Autodesk Inventor part; units mm, degrees
ref_plane "YZ Plane" through (0, 0, 0) normal (1, 0, 0) x (0, 1, 0)
ref_plane "XZ Plane" through (0, 0, 0) normal (0, 1, 0) x (-1, 0, 0)
ref_plane "XY Plane" through (0, 0, 0) normal (0, 0, 1) x (1, 0, 0)
ref_plane "작업 평면1" through (44.8, 0, -17) normal (-1, 0, 0) x (0, 0, 1)
sketch "스케치2" plane through (44.8, 0, -17) normal (-1, 0, 0) x (0, 0, 1)
  arc A0 (-19.5808, 6.2636) -> (-20.1, 4.5766) centre (-17.1, 4.5766) ccw
  line L0 (-20.1, -39.6766) -> (-20.1, 4.5766)
  arc A1 (-20.1, -39.6766) -> (-19.5808, -41.3636) centre (-17.1, -39.6766) ccw
  line L1 (-15.8929, -46.7869) -> (-19.5808, -41.3636)
  arc A2 (-15.8929, -46.7869) -> (-13.4121, -48.1) centre (-13.4121, -45.1) ccw
  line L2 (13.4121, -48.1) -> (-13.4121, -48.1)
  arc A3 (13.4121, -48.1) -> (15.8929, -46.7869) centre (13.4121, -45.1) ccw
  line L3 (19.5808, -41.3636) -> (15.8929, -46.7869)
  arc A4 (19.5808, -41.3636) -> (20.1, -39.6766) centre (17.1, -39.6766) ccw
  line L4 (20.1, 4.5766) -> (20.1, -39.6766)
  arc A5 (20.1, 4.5766) -> (19.5808, 6.2636) centre (17.1, 4.5766) ccw
  line L5 (15.5953, 12.1246) -> (19.5808, 6.2636)
  arc A6 (15.5953, 12.1246) -> (13.9414, 13) centre (13.9414, 11) ccw
  line L6 (7.65, 13) -> (13.9414, 13)
  arc A7 (9.15, 11.5) -> (7.65, 13) centre (7.65, 11.5) ccw
  line L7 (9.15, 11.5) -> (9.15, 10)
  arc A8 (9.15, 10) -> (11.5, 7.65) centre (11.5, 10) ccw
  line L8 (11.5, 7.65) -> (13.5, 7.65)
  arc A9 (14.5, 6.65) -> (13.5, 7.65) centre (13.5, 6.65) ccw
  line L9 (14.5, 6.65) -> (14.5, -36.15)
  arc A10 (13.5, -37.15) -> (14.5, -36.15) centre (13.5, -36.15) ccw
  line L10 (13.5, -37.15) -> (11.5, -37.15)
  arc A11 (11.5, -37.15) -> (9.15, -39.5) centre (11.5, -39.5) ccw
  line L11 (9.15, -39.5) -> (9.15, -41.5)
  arc A12 (8.15, -42.5) -> (9.15, -41.5) centre (8.15, -41.5) ccw
  line L12 (8.15, -42.5) -> (-8.15, -42.5)
  arc A13 (-9.15, -41.5) -> (-8.15, -42.5) centre (-8.15, -41.5) ccw
  line L13 (-9.15, -41.5) -> (-9.15, -39.5)
  arc A14 (-9.15, -39.5) -> (-11.5, -37.15) centre (-11.5, -39.5) ccw
  line L14 (-11.5, -37.15) -> (-13.5, -37.15)
  arc A15 (-14.5, -36.15) -> (-13.5, -37.15) centre (-13.5, -36.15) ccw
  line L15 (-14.5, -36.15) -> (-14.5, 6.65)
  arc A16 (-13.5, 7.65) -> (-14.5, 6.65) centre (-13.5, 6.65) ccw
  line L16 (-13.5, 7.65) -> (-11.5, 7.65)
  arc A17 (-11.5, 7.65) -> (-9.15, 10) centre (-11.5, 10) ccw
  line L17 (-9.15, 10) -> (-9.15, 11.5)
  arc A18 (-7.65, 13) -> (-9.15, 11.5) centre (-7.65, 11.5) ccw
  line L18 (-13.9414, 13) -> (-7.65, 13)
  arc A19 (-13.9414, 13) -> (-15.5953, 12.1246) centre (-13.9414, 11) ccw
  line L19 (-19.5808, 6.2636) -> (-15.5953, 12.1246)
  circle A20 centre (17.3, 4) radius 1.35
  circle A21 centre (17.3, -18) radius 1.35
  circle A22 centre (11, -45.3) radius 1.35
  circle A23 centre (-17.3, 4) radius 1.35
  circle A24 centre (-17.3, -18) radius 1.35
  circle A25 centre (-11, -45.3) radius 1.35
  circle A26 centre (17.3, -40) radius 1.35
  circle A27 centre (-17.3, -40) radius 1.35
  line L20 (17.3, -19.35) -> (17.3, 5.35)
  line L21 (20.1, 4.5766) -> (20.1, 6.65)
  line L22 (20.1, 6.65) -> (14.5, 6.65)
  line L23 (17.3, -7) -> (20.1, -7)
  arc A28 (19.5808, -20.2636) -> (20.1, -18.5766) centre (17.1, -18.5766) ccw
  line L24 (20.1, -18.5766) -> (20.1, -20.65)
  line L25 (20.1, -20.65) -> (14.5, -20.65)
  line L26 (20.1, -20.65) -> (14.5, -20.65)
  line L27 (14.5, -20.65) -> (14.5, 6.65)
  line L28 (14.5, 6.65) -> (20.1, 6.65)
  line L29 (20.1, 6.65) -> (20.1, -20.65)
  line L30 (14.6, -36.15) -> (14.6, 6.65)
  arc A29 (14.6, 6.65) -> (13.5, 7.75) centre (13.5, 6.65) ccw
  line L31 (13.5, 7.75) -> (11.5, 7.75)
  arc A30 (9.25, 10) -> (11.5, 7.75) centre (11.5, 10) ccw
  line L32 (9.25, 10) -> (9.25, 11.5)
  arc A31 (9.25, 11.5) -> (8.4246, 12.9) centre (7.65, 11.5) ccw
  line L33 (8.4246, 12.9) -> (13.9414, 12.9)
  arc A32 (15.5126, 12.0684) -> (13.9414, 12.9) centre (13.9414, 11) ccw
  line L34 (15.5126, 12.0684) -> (19.4981, 6.2073)
  arc A33 (20, 4.5766) -> (19.4981, 6.2073) centre (17.1, 4.5766) ccw
  line L35 (20, 4.5766) -> (20, -39.6766)
  arc A34 (19.4981, -41.3073) -> (20, -39.6766) centre (17.1, -39.6766) ccw
  line L36 (19.4981, -41.3073) -> (15.8102, -46.7307)
  arc A35 (13.4121, -48) -> (15.8102, -46.7307) centre (13.4121, -45.1) ccw
  line L37 (13.4121, -48) -> (-13.4121, -48)
  arc A36 (-15.8102, -46.7307) -> (-13.4121, -48) centre (-13.4121, -45.1) ccw
  line L38 (-15.8102, -46.7307) -> (-19.4981, -41.3073)
  arc A37 (-20, -39.6766) -> (-19.4981, -41.3073) centre (-17.1, -39.6766) ccw
  line L39 (-20, -39.6766) -> (-20, 4.5766)
  arc A38 (-19.4981, 6.2073) -> (-20, 4.5766) centre (-17.1, 4.5766) ccw
  line L40 (-19.4981, 6.2073) -> (-15.5126, 12.0684)
  arc A39 (-13.9414, 12.9) -> (-15.5126, 12.0684) centre (-13.9414, 11) ccw
  line L41 (-13.9414, 12.9) -> (-8.4246, 12.9)
  arc A40 (-8.4246, 12.9) -> (-9.25, 11.5) centre (-7.65, 11.5) ccw
  line L42 (-9.25, 11.5) -> (-9.25, 10)
  arc A41 (-11.5, 7.75) -> (-9.25, 10) centre (-11.5, 10) ccw
  line L43 (-11.5, 7.75) -> (-13.5, 7.75)
  arc A42 (-13.5, 7.75) -> (-14.6, 6.65) centre (-13.5, 6.65) ccw
  line L44 (-14.6, 6.65) -> (-14.6, -36.15)
  arc A43 (-14.6, -36.15) -> (-13.5, -37.25) centre (-13.5, -36.15) ccw
  line L45 (-13.5, -37.25) -> (-11.5, -37.25)
  arc A44 (-9.25, -39.5) -> (-11.5, -37.25) centre (-11.5, -39.5) ccw
  line L46 (-9.25, -39.5) -> (-9.25, -41.5)
  arc A45 (-9.25, -41.5) -> (-8.15, -42.6) centre (-8.15, -41.5) ccw
  line L47 (-8.15, -42.6) -> (8.15, -42.6)
  arc A46 (8.15, -42.6) -> (9.25, -41.5) centre (8.15, -41.5) ccw
  line L48 (9.25, -41.5) -> (9.25, -39.5)
  arc A47 (11.5, -37.25) -> (9.25, -39.5) centre (11.5, -39.5) ccw
  line L49 (11.5, -37.25) -> (13.5, -37.25)
  arc A48 (13.5, -37.25) -> (14.6, -36.15) centre (13.5, -36.15) ccw
  line L50 (20, 4.5766) -> (20, 6.65)
  line L51 (17, 8.5) -> (17, -44.6)
  line L52 (17, 8.5) -> (17, -44.6)
  point P0 (17, 0)
  point P1 (17.3, -18)
  point P2 (14.6, -20.65)
  point P3 (20, -20.65)
  dimension "d3" = 0.1
extrude "돌출2" add sketch "스케치2" along normal blind 24.6 contours L25 L51 A21 L20 L23 L35 | L25 L30 L22 L51 A20 A21 | L23 L20 A20 L51 L22 L34 A33 L35 | L50 A33 L34 L22 L5 A5 | A5 L5 L22 L50 | L20 A21 L51 A20
sketch "스케치3" plane through (20.2, 0, -17) normal (-1, 0, 0) x (0, 0, 1)
  line L0 (17, 8.5) -> (17, -44.6)
  line L1 (14.6, -20.65) -> (20, -20.65)
  line L2 (20, -20.65) -> (20, 6.65)
  line L3 (17, -20.65) -> (20, -20.65)
  line L4 (20, -20.65) -> (20, 6.65)
  line L5 (20, 6.65) -> (17, 6.65)
  line L6 (17, 6.65) -> (17, -20.65)
  line L7 (17.1, 8.5) -> (17.1, -44.6)
  point P0 (17, 0)
  point P1 (17.1, 6.65)
  point P2 (17.1, -20.65)
  dimension "d6" = 0.1
extrude "돌출3" add sketch "스케치3" along normal blind 5.6 contours L5 L2 L1 L7
sketch "스케치4" plane through (44.8, -20.65, 3) normal (0, 0, 1) x (1, 0, 0)
  line L0 (-31.3, -19.1) -> (-33.3, -19.1)
  arc A0 (-33.3, -19.1) -> (-35.55, -21.35) centre (-33.3, -21.35) ccw
  line L1 (-35.55, -21.35) -> (-35.55, -23.35)
  arc A1 (-36.55, -24.35) -> (-35.55, -23.35) centre (-36.55, -23.35) ccw
  line L2 (-36.55, -24.35) -> (-53.05, -24.35)
  arc A2 (-54.05, -23.35) -> (-53.05, -24.35) centre (-53.05, -23.35) ccw
  line L3 (-54.05, -23.35) -> (-54.05, -21.35)
  arc A3 (-54.05, -21.35) -> (-56.3, -19.1) centre (-56.3, -21.35) ccw
  line L4 (-56.3, -19.1) -> (-58.3, -19.1)
  arc A4 (-59.3, -18.1) -> (-58.3, -19.1) centre (-58.3, -18.1) ccw
  line L5 (-59.3, -18.1) -> (-59.3, 28.9)
  arc A5 (-58.3, 29.9) -> (-59.3, 28.9) centre (-58.3, 28.9) ccw
  line L6 (-58.3, 29.9) -> (-56.3, 29.9)
  arc A6 (-56.3, 29.9) -> (-54.05, 32.15) centre (-56.3, 32.15) ccw
  line L7 (-54.05, 32.15) -> (-54.05, 35.15)
  line L8 (-59.8, 35.15) -> (-54.05, 35.15)
  line L9 (-64.9, 29.15) -> (-59.8, 35.15)
  line L10 (-64.9, -23.95) -> (-64.9, 29.15)
  line L11 (-59.8, -29.95) -> (-64.9, -23.95)
  line L12 (-29.8, -29.95) -> (-59.8, -29.95)
  line L13 (-24.7, -23.95) -> (-29.8, -29.95)
  line L14 (-24.7, 29.15) -> (-24.7, -23.95)
  line L15 (-29.8, 35.15) -> (-24.7, 29.15)
  line L16 (-35.55, 35.15) -> (-29.8, 35.15)
  line L17 (-35.55, 35.15) -> (-35.55, 32.15)
  arc A7 (-35.55, 32.15) -> (-33.3, 29.9) centre (-33.3, 32.15) ccw
  line L18 (-33.3, 29.9) -> (-31.3, 29.9)
  arc A8 (-30.3, 28.9) -> (-31.3, 29.9) centre (-31.3, 28.9) ccw
  line L19 (-30.3, 28.9) -> (-30.3, -18.1)
  arc A9 (-31.3, -19.1) -> (-30.3, -18.1) centre (-31.3, -18.1) ccw
  circle A10 centre (-27.5, 24.65) radius 1.35
  circle A11 centre (-27.5, 2.65) radius 1.35
  circle A12 centre (-33.8, -27.15) radius 1.35
  circle A13 centre (-62.1, 24.65) radius 1.35
  circle A14 centre (-62.1, 2.65) radius 1.35
  circle A15 centre (-55.8, -27.15) radius 1.35
  circle A16 centre (-27.5, -19.35) radius 1.35
  circle A17 centre (-62.1, -19.35) radius 1.35
  point P0 (-44.8, 20.65)
extrude "돌출4" cut sketch "스케치4" against normal up to next contours A10 | A11
sketch "스케치5" plane through (44.8, -20.65, 3) normal (0, 0, 1) x (1, 0, 0)
  line L0 (-5.275, 23.4) -> (2.4, 23.4)
  line L1 (-5.275, 25.9) -> (2.4, 25.9)
  line L2 (-5.275, 23.4) -> (-5.275, 25.9)
  line L3 (-5.275, 24.65) -> (2.4, 24.65)
  line L4 (-5.275, 24.65) -> (-3.075, 24.65)
  line L5 (-3.075, 24.65) -> (-3.075, 22.05)
  line L6 (-3.075, 22.05) -> (-5.275, 22.05)
  line L7 (-5.275, 22.05) -> (-5.275, 24.65)
  line L8 (-3.075, 24.65) -> (-3.075, 27.25)
  line L9 (-3.075, 27.25) -> (-5.275, 27.25)
  line L10 (-5.275, 27.25) -> (-5.275, 24.65)
  line L11 (0, 27.3) -> (-30.2, 27.3)
  line L12 (-3.075, 27.25) -> (-5.275, 27.25)
  line L13 (-5.275, 27.25) -> (-5.275, 27.3)
  line L14 (-5.275, 27.3) -> (-3.075, 27.3)
  line L15 (-3.075, 27.3) -> (-3.075, 27.25)
  circle A0 centre (-27.5, 24.65) radius 1.35
  circle A1 centre (-27.5, 2.65) radius 1.35
  line L16 (0, 0) -> (0, 27.3)
  line L17 (0, 27.3) -> (-30.2, 27.3)
  line L18 (-30.2, 0) -> (-30.2, 27.3)
  line L19 (0, 0) -> (-30.2, 0)
  line L20 (0, 13.65) -> (-30.2, 13.65)
  line L21 (-5.275, 3.9) -> (-5.275, 1.4)
  line L22 (-5.275, 2.65) -> (-3.075, 2.65)
  line L23 (-3.075, 2.65) -> (-3.075, 5.25)
  line L24 (-3.075, 5.25) -> (-5.275, 5.25)
  line L25 (-5.275, 5.25) -> (-5.275, 2.65)
  line L26 (-3.075, 2.65) -> (-3.075, 0.05)
  line L27 (-3.075, 0.05) -> (-5.275, 0.05)
  line L28 (-5.275, 0.05) -> (-5.275, 2.65)
  line L29 (-3.075, 0.05) -> (-5.275, 0.05)
  line L30 (-5.275, 0.05) -> (-5.275, 0)
  line L31 (-5.275, 0) -> (-3.075, 0)
  line L32 (-3.075, 0) -> (-3.075, 0.05)
  point P0 (-44.8, 20.65)
  point P1 (-3.075, 27.3)
  point P2 (-5.275, 27.25)
  point P3 (-5.275, 25.9)
  point P4 (-5.275, 23.4)
  point P5 (-5.275, 0.05)
  point P6 (-5.275, 0)
  point P7 (-3.075, 0)
  point P8 (-5.275, 3.9)
  point P9 (-5.275, 1.4)
  dimension "d11" = 2.2
  dimension "d12" = 2.6
extrude "돌출5" cut sketch "스케치5" against normal blind 10 contours L2 L3 L5 L0 | L0 L5 L6 L7 | L2 L1 L8 L3 | L10 L9 L8 L1 | L13 L11 L15 L9 | L19 L30 L27 L32 | L27 L28 L21 L22 L26 | L22 L21 L25 L24 L23
properties part number "64-106_connect"
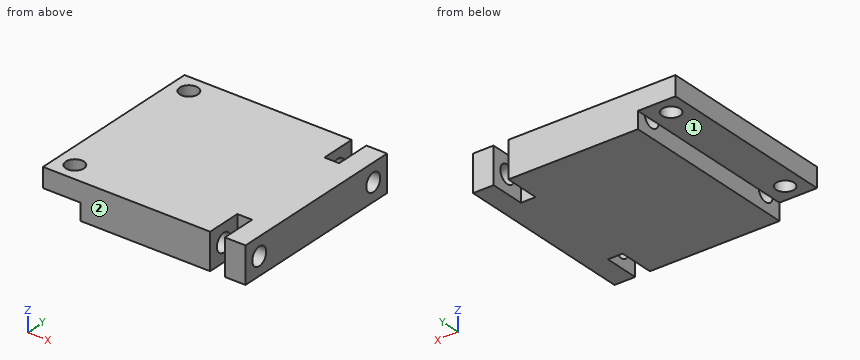
Read the model definition and answer for the solid it produces. Units are mm, in the model's axes. Face numbers are marked on the shaded views. A direction names the side the tool comes from. Give positions to 0.01 mm unless a question says otherwise; leave off trailing zeros. Order: outer loops, then holes, each group sorted by start corner. A loop starts at its lowest first (then second) coordinate and runs counter-clockwise, first axis right, second up.
(1) Find section C-C (z = 2.3). Give the vertices of the cut face in (x, y) (3 decimals).
(2) Straight lines are drawn through the part: L1, parallel to Y at x = 17.3, z = 1.55; L2, parallel to X at y = -17.25, z = -1.6 (3 decimals); L3, parallel to Y at x = 27.5, z = -0.45. For each, find the intervals that lie inside material, in ascending order.
(3) For the marked faces 1 and 2, determine the directions among +Z, -Z, +X, -X, +Y, -Y from which every point of the face is accessible in a straight line to the end or side of a thin tool.
(4) Find section B-B (x = 17.3). Give the vertices of the cut face in (y, z), plus the area to 3 significant figures.
(5) Given pin 1 (0.8 mm diameter, centred on y = -13, z = -1, fed in from -X); pin 2 (0.8 mm diameter, centred on y = -18.5, z = 1, fed in from +X), each flat-ended and moving along its own axis, determine where each tip first touches the part or whether it passes through.
(6) Find section D-D (x = 24.5). Give the vertices of the cut face in (y, z), plus the area to 3 significant figures.
(7) Find section A-A (y = -18). Give the vertices of the cut face in (x, z) (3 decimals).
Result sheet:
1. outline: (14.6, -20.65) - (39.525, -20.65) - (39.525, -15.4) - (41.725, -15.4) - (41.725, -20.65) - (44.8, -20.65) - (44.8, 6.65) - (41.725, 6.65) - (41.725, 1.4) - (39.525, 1.4) - (39.525, 6.65) - (14.6, 6.65) - close; hole circle Ø2.7 at (17.3, -18); hole circle Ø2.7 at (17.3, 4)
2. L1: y = -20.65 to -19.35, -16.65 to 2.65, 5.35 to 6.65
2. L2: x = 20.2 to 39.525, 41.725 to 44.8
2. L3: y = -20.65 to -19.12, -16.88 to 2.88, 5.12 to 6.65
3. face 1: -Z, -X, +Y, -Y
3. face 2: +Z, -Z, +X, -X, -Y
4. outline: (-20.65, 0.1) - (-19.35, 0.1) - (-19.35, 3) - (-20.65, 3) - close; (-16.65, 0.1) - (2.65, 0.1) - (2.65, 3) - (-16.65, 3) - close; (5.35, 0.1) - (6.65, 0.1) - (6.65, 3) - (5.35, 3) - close
4. area: 63.5 mm2
5. pin 1: stops at x = 20.2
5. pin 2: stops at x = 20.2
6. outline: (-20.65, -2.4) - (6.65, -2.4) - (6.65, 3) - (-20.65, 3) - close; hole circle Ø2.7 at (-18, 0.3); hole circle Ø2.7 at (4, 0.3)
6. area: 136 mm2
7. outline: (14.6, 0.1) - (15.95, 0.1) - (15.95, 3) - (14.6, 3) - close; (18.65, 0.1) - (20.2, 0.1) - (20.2, 1.65) - (39.525, 1.65) - (39.525, 3) - (18.65, 3) - close; (20.2, -2.4) - (39.525, -2.4) - (39.525, -1.05) - (20.2, -1.05) - close; (41.725, -2.4) - (44.8, -2.4) - (44.8, -1.05) - (41.725, -1.05) - close; (41.725, 1.65) - (44.8, 1.65) - (44.8, 3) - (41.725, 3) - close
